The listing builds one solid part. Answer for the finished solid, in the listing's coordinates (mm). Face numbers are marked on the shaded views. Give positions to 0.01 mm unless a question says otherwise; leave off trailing zeros. Loops run counter-clockwise (first coordinate to the right, second up) from the corner with the lowest first, then second, coordinate; pieces in that order, holes last. Notation, with made-up numbers: (43, -22) - (76, -22) arc R8 cw to (76, -17) - close; hole circle Ø8 at (-26.5, 36.5). An arc over 180 degrees is marked (long way). One line per item, written item: value. Start each with the question number.
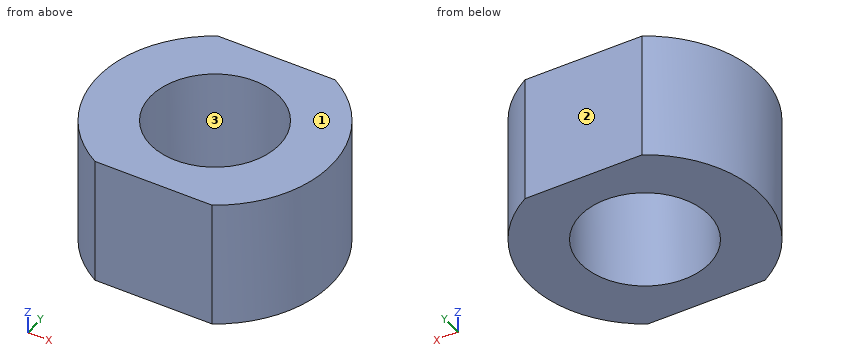
from build123d import *

# Parameters (mm, degrees)
ESQUISSE1_R             = 6.35
BOSS_EXTRU_1_DEPTH      = 7
ESQUISSE2_R             = 3.5
ENL_V_MAT_EXTRU_1_DEPTH = 7
ESQUISSE3_W             = 10.71653065
ESQUISSE3_H             = 1.876238016
ENL_V_MAT_EXTRU_2_DEPTH = 12.386175829


with BuildPart() as part:
    # Esquisse1 → Boss.-Extru.1 (new body)
    with BuildSketch(Plane.XY):
        Circle(ESQUISSE1_R)
    extrude(amount=BOSS_EXTRU_1_DEPTH)

    # Esquisse2 → Enlèv. mat.-Extru.1 (cut)
    with BuildSketch(Plane.XY.offset(7)):
        Circle(ESQUISSE2_R)
    extrude(amount=-ENL_V_MAT_EXTRU_1_DEPTH, mode=Mode.SUBTRACT)

    # Esquisse3 → Enlèv. mat.-Extru.2 (cut, through all)
    with BuildSketch(Plane.XY.offset(7)):
        with Locations((0.338060904, 6.438119008)):
            Rectangle(ESQUISSE3_W, ESQUISSE3_H)
        with Locations((0.338060904, -6.438119008)):
            Rectangle(ESQUISSE3_W, ESQUISSE3_H)
    extrude(amount=-ENL_V_MAT_EXTRU_2_DEPTH, mode=Mode.SUBTRACT)


solid = part.part
1. Find the intervals of material crossed by L1, parallel to Y at x = 0, z = 4; L2, parallel to Y at x = 2.5, z = 6.75; L3, parallel to X at y = 0.75, z = 5.5, in increasing order. Write a range as [from, to].
2. A cutting plane is placed at A-A (y = 0). Determine the outline of the cut face in (x, z).
3. Determine the mould class of the marked faces 1, 2 and 3 for opening direction Y: released by +Y, released by -Y, zero draft, split by the parting line, or undercut.
4. A cutting plane is placed at C-C (z = 5). Determine the outline of the cut face in (x, y), plus the area to 3 significant figures.
5. A cutting plane is placed at D-D (y = 4.5). Determine the outline of the cut face in (x, z).
6. A cutting plane is placed at B-B (x = 0). Determine the outline of the cut face in (y, z), plus the area to 3 significant figures.
Results below:
1. L1: y = [-5.5, -3.5], [3.5, 5.5]
1. L2: y = [-5.5, -2.45], [2.45, 5.5]
1. L3: x = [-6.31, -3.42], [3.42, 6.31]
2. outline: (-6.35, 0) - (-3.5, 0) - (-3.5, 7) - (-6.35, 7) - close; (3.5, 0) - (6.35, 0) - (6.35, 7) - (3.5, 7) - close
3. face 1: zero draft
3. face 2: released by +Y
3. face 3: undercut
4. outline: (-3.17, -5.5) - (3.17, -5.5) arc R6.35 ccw to (3.17, 5.5) - (-3.17, 5.5) arc R6.35 ccw to start; hole circle Ø7 at (0, 0)
4. area: 80.9 mm^2
5. outline: (-4.48, 0) - (4.48, 0) - (4.48, 7) - (-4.48, 7) - close
6. outline: (-5.5, 0) - (-3.5, 0) - (-3.5, 7) - (-5.5, 7) - close; (3.5, 0) - (5.5, 0) - (5.5, 7) - (3.5, 7) - close
6. area: 28.0 mm^2
